Can you work these out from the drawing? Everything is in mm from the part's minimum corner. A direction names the side the tool comes from. Round coordinates to 2 decimals unless told otherwise and drop trailing zeros. Loops run counter-clockwise (first coordinate to the right, second up) from the corner with the lowest first, then second, coordinate; pieces in that order, holes last. Notation, with made-up numbers: M -18,43 L 22,43 A17 ccw 22,62 Z; hole C 44.5,-10.75 d6. An arc over 180 degrees is marked long. Use a Markdown table: item, result.
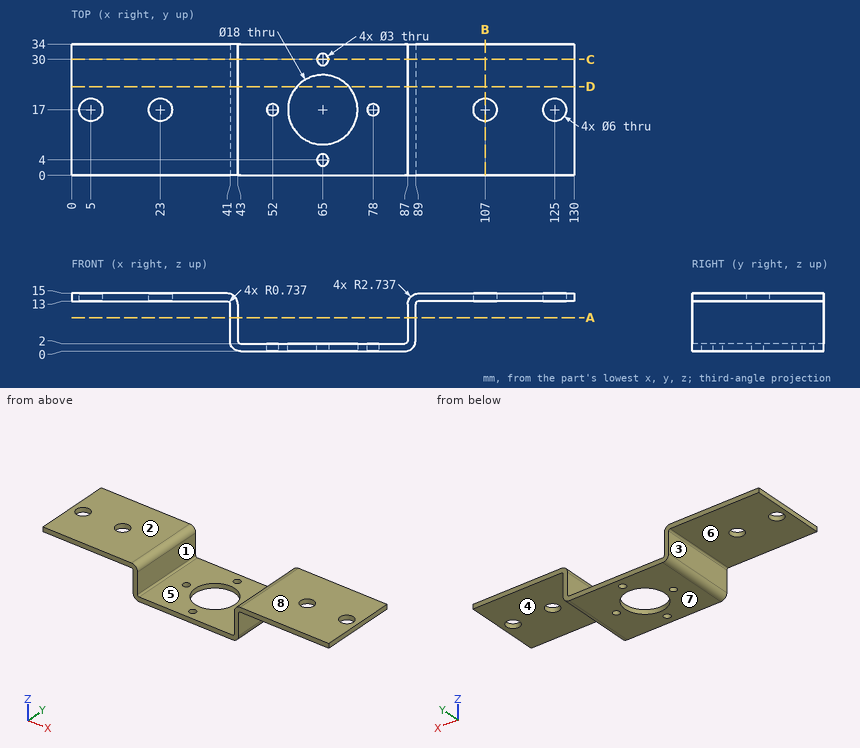
Q1. We'd pull the mould along X, two halves only. Please class the marked faces 1, 2 and 3: pulls with the +X half, pulls with the -X half, needs draft (parallel to the pull), parting line crosses it, or undercut.
Return value:
| item | result |
|---|---|
| face 1 | undercut |
| face 2 | needs draft |
| face 3 | pulls with the -X half |
Q2. Imagine slicing it at A-A, the plane z = 8.75. Please give me the cut outline in (x, y).
Return value:
| item | result |
|---|---|
| outline | M 41,0 L 43,0 L 43,34 L 41,34 Z; M 87,0 L 89,0 L 89,34 L 87,34 Z |
Q3. Will these pins go through, and if not, where does the flat tip stop? P1, Ø3, axis at y = 10.5, z = 6, coming from the -X side; P2, Ø8, axis at x = 65.5, z = 9.5, coming from the +Y side; P3, Ø5, axis at x = 79, y = 5.5, coming from the +Z side; P4, Ø9.5, axis at x = 107, y = 17, coming from the -Z side.
Return value:
| item | result |
|---|---|
| P1 | stops at x = 41 |
| P2 | passes through |
| P3 | stops at z = 2 |
| P4 | stops at z = 13 |
Q4. Imagine slicing it at C-C, the plane y = 30. Please give me the cut outline in (x, z).
Return value:
| item | result |
|---|---|
| outline | M 0,13 L 40.26,13 A0.74 cw 41,12.26 L 41,2.74 A2.74 ccw 43.74,0 L 63.5,0 L 63.5,2 L 43.74,2 A0.74 cw 43,2.74 L 43,12.26 A2.74 ccw 40.26,15 L 0,15 Z; M 66.5,0 L 86.26,0 A2.74 ccw 89,2.74 L 89,12.26 A0.74 cw 89.74,13 L 130,13 L 130,15 L 89.74,15 A2.74 ccw 87,12.26 L 87,2.74 A0.74 cw 86.26,2 L 66.5,2 Z |
Q5. I need wall thicknesses on line 1 (X direction, y = 20.5, z = 3.5); line 2 (Y direction, x = 65, z = 1.25); line 3 (Y direction, x = 23, z = 13.85). Which ranges of each line are inside material? Lowest first, please. Write a range as from..to.
Return value:
| item | result |
|---|---|
| line 1 | x = 41..43, 87..89 |
| line 2 | y = 0..2.5, 5.5..8, 26..28.5, 31.5..34 |
| line 3 | y = 0..14, 20..34 |
Q6. Imagine slicing it at D-D, the plane y = 23. Please give me the cut outline in (x, z), then the cut area to 3 significant figures.
Return value:
| item | result |
|---|---|
| outline | M 0,13 L 40.26,13 A0.74 cw 41,12.26 L 41,2.74 A2.74 ccw 43.74,0 L 58.29,0 L 58.29,2 L 43.74,2 A0.74 cw 43,2.74 L 43,12.26 A2.74 ccw 40.26,15 L 0,15 Z; M 71.71,0 L 86.26,0 A2.74 ccw 89,2.74 L 89,12.26 A0.74 cw 89.74,13 L 130,13 L 130,15 L 89.74,15 A2.74 ccw 87,12.26 L 87,2.74 A0.74 cw 86.26,2 L 71.71,2 Z |
| area | 279 mm^2 |
Q7. Imagine slicing it at B-B, the plane x = 107. Please give me the cut outline in (y, z).
Return value:
| item | result |
|---|---|
| outline | M 0,13 L 14,13 L 14,15 L 0,15 Z; M 20,13 L 34,13 L 34,15 L 20,15 Z |
Q8. For the marked faces 4, 5, 6, 7 and 8, which set-ups out of +Z, -Z, +X, -X, +Y, -Y let a thin tool reach every point of the face, with its end or its side?
Return value:
| item | result |
|---|---|
| face 4 | -Z, +X, +Y, -Y |
| face 5 | +Z, +Y, -Y |
| face 6 | -Z, -X, +Y, -Y |
| face 7 | -Z, +X, -X, +Y, -Y |
| face 8 | +Z, +X, -X, +Y, -Y |
